from build123d import *

# Parameters (mm, degrees)
F1_DEPTH = 10
F2_DEPTH = 10


with BuildPart() as f1:
    # F0 (on Front) → F1 (new body)
    with BuildSketch(Plane.XZ):
        Polygon((0, 26.44526), (0, 43.04029), (-10, 43.04029), (-10, -31.95971), (0, -31.95971), align=None)
    extrude(amount=F1_DEPTH)

    # F0 (on Front) → F2 (join)
    with BuildSketch(Plane.XZ):
        Polygon((0, 26.44526), (0, 43.04029), (-10, 43.04029), (-10, -31.95971), (0, -31.95971), align=None)
        Polygon((23.582859, 34.742775), (0, 43.04029), (0, 26.44526), align=None)
    extrude(amount=F2_DEPTH)


solid = f1.part
Could you check a few things on this model? Use its own coordinates, in mm. A direction names the side the tool comes from. Give positions to 0.01 mm unless a question says otherwise; leave off trailing zeros. Order: outer loops, then holes, each group sorted by start corner. A loop starts at its lowest first (then second) coordinate and runs counter-clockwise, first axis right, second up. Notation, with made-up numbers: (88.25, 26) -> (106.25, 26) arc R27 ccw to (106.25, 58) -> close; hole circle Ø10 at (-34.5, 77.25). An arc over 180 degrees is marked (long way). Return JSON: item names as keys, results as strings.
1. I need wall thicknesses on line 1 (X direction, y = -0.75, z = 12.5); line 2 (Z direction, x = 15.5, y = -9); line 3 (Z direction, x = 3.5, y = -5). Which ranges of each line are inside material? Lowest first, please. Write a range as from..to.
Answer list:
{"line 1": "x = -10..0", "line 2": "z = 31.9..37.59", "line 3": "z = 27.68..41.81"}
2. On a 3-axis mill with a long thin cutter (end or side, diameter ignored), from which of +Z, -Z, +X, -X, +Y, -Y can I reach the whole of each face in a straight line? I mean faces 1 (the flat face through (0, -5, -3)), 2 (the flat face through (-5, -5, 43.04)). Say none if no direction works.
Answer list:
{"face 1": "-Z, +X, +Y, -Y", "face 2": "+Z, +X, -X, +Y, -Y"}
3. Imagine slicing it at A-A on y = -5.5. List the corners of the cut face in (x, z) for me.
Answer list:
{"outline": "(-10, -31.96) -> (0, -31.96) -> (0, 26.45) -> (23.58, 34.74) -> (0, 43.04) -> (-10, 43.04) -> close"}
4. Imagine slicing it at C-C on x = 14.5. List the corners of the cut face in (y, z) for me.
Answer list:
{"outline": "(-10, 31.55) -> (0, 31.55) -> (0, 37.94) -> (-10, 37.94) -> close"}
5. Imagine slicing it at B-B on z = -6.5. List the corners of the cut face in (x, y) for me.
Answer list:
{"outline": "(-10, -10) -> (0, -10) -> (0, 0) -> (-10, 0) -> close"}
6. For pin 1 Ø10 at (x, z) = (9, 11.5) entering from +Y; pin 2 Ø8 at (x, z) = (12, 26.5) entering from -Y; pin 3 Ø2 at (x, y) = (16, -8) entering from +Z; pin 4 Ø2 at (y, z) = (-7, -10.5) entering from +X, each with a flat end and sliding along its axis, tell me the tip position at first contact or that it passes through.
Answer list:
{"pin 1": "passes through", "pin 2": "stops at y = -10", "pin 3": "stops at z = 37.76", "pin 4": "stops at x = 0"}
